Can you work these out from the model? Positions are in its coordinate system, mm. Give positions to 0.01 mm unless a question says otherwise; leave off trailing zeros. Loops run counter-clockwise (first coordinate to the right, second up) from the corner with the lowest first, then second, coordinate; pieces in that order, holes last. Notation, with made-up numbers: (67, 86) - (96, 86) arc R17 ccw to (96, 105) - close; hole circle Ø9 at (-31.5, 88). An arc over 180 degrees is marked (long way). Answer as a JSON object with one key per item and string values.
```python
from build123d import *

# Parameters (mm, degrees)
EXTRUDE1_DEPTH       = 914.4
MIRROR2_COPY_1_DEPTH = 914.4


with BuildPart() as part:
    # Sketch1 → Extrude1 (new, symmetric)
    with BuildSketch(Plane.XY):
        Polygon((-25.4, -0.6604), (-5.159375, -0.9906), (0, -0.79375), (0, 0), (-25.4, 0), align=None)
    extrude1 = extrude(amount=EXTRUDE1_DEPTH, both=True)

    # Mirror1: Extrude1 across plane
    add(extrude1.mirror(Plane(origin=(0, 0, 0), x_dir=(0, 0, 1), z_dir=(1, 0, 0))))

    # Mirror2: Extrude1 across plane
    add(extrude1.mirror(Plane.ZX))

    # Mirror2 copy 1 sketch → Mirror2 copy 1 (add, symmetric)
    with BuildSketch(Plane(origin=(0, 0, 0), x_dir=(-1, 0, 0), z_dir=(0, 0, 1))):
        Polygon((-25.4, -0.6604), (-5.159375, -0.9906), (0, -0.79375), (0, 0), (-25.4, 0), align=None)
    extrude(amount=MIRROR2_COPY_1_DEPTH, both=True)


solid = part.part
```
1) Imagine slicing it at A-A on z = 793.5. Write out the boundary of the cut face in (x, y), and give its area (3 significant figures).
Check sheet entries:
{"outline": "(-25.4, -0.66) - (-5.16, -0.99) - (0, -0.79) - (5.16, -0.99) - (25.4, -0.66) - (25.4, 0.66) - (5.16, 0.99) - (0, 0.79) - (-5.16, 0.99) - (-25.4, 0.66) - close", "area": "85.2 mm2"}
2) I need wall thicknesses on L1, parallel to Y at x = 21, z = -574; L2, parallel to Y at x = 1, z = 783.5. Which ranges of each line are inside material? Lowest first, please.
Check sheet entries:
{"L1": "-0.73 to 0.73", "L2": "-0.83 to 0.83"}
3) I'm going to push flat-ended pins straight in: P1, Ø12, axis at x = -11.5, z = -229.5, coming from the -Y side; P2, Ø1.5, axis at x = 19, z = 56.5, coming from the +Y side. Where does each tip first touch, or does it pass through?
Check sheet entries:
{"P1": "y = -0.99", "P2": "y = 0.78"}
4) Imagine slicing it at B-B on x = -16.5. Write out the boundary of the cut face in (y, z).
Check sheet entries:
{"outline": "(-0.81, -914.4) - (0.81, -914.4) - (0.81, 914.4) - (-0.81, 914.4) - close"}
